from build123d import *

# Parameters (mm, degrees)
SKETCH1_W          = 8
SKETCH1_H          = 3
CUT_EXTRUDE2_DEPTH = 2.31


with BuildPart() as part:
    # Sketch1 → Revolve1 (revolve)
    with BuildSketch(Plane(origin=(0, 0, 0), x_dir=(0, 0, -1), z_dir=(1, 0, 0))):
        with Locations((7.3, 1.5)):
            Rectangle(SKETCH1_W, SKETCH1_H)
    revolve(axis=Axis((0, 0, -11.3), (0, 0, 1)))

    # Sketch7 → Revolve2 (revolve)
    with BuildSketch(Plane(origin=(0, 0, 0), x_dir=(0, 0, -1), z_dir=(1, 0, 0)), mode=Mode.PRIVATE) as revolve2_sk:
        with BuildLine():
            Line((2.805, 5.25), (3.3, 5.25))
            Line((3.3, 5.25), (3.3, 0))
            Line((3.3, 0), (0, 0))
            Line((0, 0), (0, 3))
            ThreePointArc((0, 3), (1.216479019, 4.356906156), (2.805, 5.25))
        make_face()
    revolve(revolve2_sk.sketch.rotate(Axis((0, 0, 0), (0, 0, -1)), 180), axis=Axis((0, 0, 0), (0, 0, -1)))

    # Sketch5 → Cut-Extrude2 (cut)
    with BuildSketch(Plane.XY):
        Polygon((2, -1.154700538), (2, 1.154700538), (0, 2.309401077), (-2, 1.154700538), (-2, -1.154700538), (0, -2.309401077), align=None)
    extrude(amount=-CUT_EXTRUDE2_DEPTH, mode=Mode.SUBTRACT)


solid = part.part
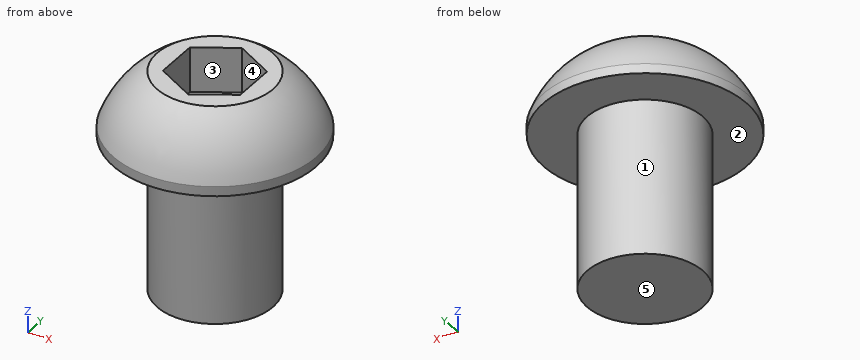
Read the model definition and answer for the solid it produces. Units are mm, in the model's axes. Face numbers are marked on the shaded views. A direction names the side the tool comes from. Coordinates: 2 decimals unless noted, no trailing zeros. Write each loop counter-clockwise with the first axis right and the second up, starting at its lowest first coordinate (ties: lowest second). Pieces come first, ordered by that corner, then holes. Notation, with made-up numbers: (47.25, 16.5) -> (80.25, 16.5) arc R35 ccw to (80.25, 55.5) -> close; hole circle Ø11 at (2, -14.5). An arc over 180 degrees is marked (long way). Return JSON: item names as keys, results as strings.
(1) Which of the six approach directions +Z, -Z, +X, -X, +Y, -Y give full straight-line access (tool end or side, diameter ignored) to the marked faces 4 and 5?
Answers below:
{"face 4": "+Z", "face 5": "-Z, +X, -X, +Y, -Y"}
(2) The part is cut by section A-A on y = 0. Give the vertices of the cut face in (x, z) (3 decimals).
Answers below:
{"outline": "(-5.25, -3.3) -> (-3, -3.3) -> (-3, -11.3) -> (3, -11.3) -> (3, -3.3) -> (5.25, -3.3) -> (5.25, -2.805) arc R5.585 ccw to (3, 0) -> (2, 0) -> (2, -2.31) -> (-2, -2.31) -> (-2, 0) -> (-3, 0) arc R5.585 ccw to (-5.25, -2.805) -> close"}
(3) Consider line 1 along X through (y, z) = (0, -6.75); line 2 along Z through (x, y) = (-1.25, -0.25); line 3 along Y through (x, z) = (-2.5, -1.5). Determine where each line is inside the solid, lowest interval first. Write a range as from..to.
Answers below:
{"line 1": "-3..3", "line 2": "-11.3..-2.31", "line 3": "-3.83..3.83"}
(4) The part is cut by section D-D on y = 2.5. Give the vertices of the cut face in (x, z) (3 decimals), then the cut area to 3 significant figures.
Answers below:
{"outline": "(-4.617, -3.3) -> (-1.658, -3.3) -> (-1.658, -11.3) -> (1.658, -11.3) -> (1.658, -3.3) -> (4.617, -3.3) -> (4.617, -2.805) arc R4.995 ccw to (1.658, 0) -> (-1.658, 0) arc R4.995 ccw to (-4.617, -2.805) -> close", "area": "51.1 mm^2"}
(5) Each of these flat-tipped pins is pushed along its axis until it touches: P1, Ø1.5, axis at x = -0.5, z = -8, coming from the +Y side; P2, Ø0.7, axis at y = -0.5, z = -0.5, coming from the -X side; P3, Ø1.2, axis at y = 0, z = -1, coming from the +X side. Where does it stop, or does it pass through?
Answers below:
{"P1": "y = 3", "P2": "x = -4.01", "P3": "x = 4.64"}
(6) For a pull along X with two mould halves and no side action, classify the marked faces 1, 2 and 3 as pulls with the +X half, pulls with the -X half, needs draft (parallel to the pull), parting line crosses it, or undercut.
Answers below:
{"face 1": "parting line crosses it", "face 2": "needs draft", "face 3": "undercut"}
(7) The part is cut by section B-B on x = -1.5. Give the vertices of the cut face in (y, z) (3 decimals).
Answers below:
{"outline": "(-5.031, -3.3) -> (-2.598, -3.3) -> (-2.598, -11.3) -> (2.598, -11.3) -> (2.598, -3.3) -> (5.031, -3.3) -> (5.031, -2.805) arc R5.38 ccw to (2.598, 0) -> (1.443, 0) -> (1.443, -2.31) -> (-1.443, -2.31) -> (-1.443, 0) -> (-2.598, 0) arc R5.38 ccw to (-5.031, -2.805) -> close"}
(8) The part is cut by section C-C on z = -9.5. Give the vertices of the cut face in (x, y).
Answers below:
{"outline": "circle Ø6 at (0, 0)"}
